Solid Edge part; units mm, degrees
sketch "Sketch1" plane through (0, 0, 0) normal (0, 0, 1) x (1, 0, 0)
  line L0 (-65, 148.37) -> (-65, 118.37)
  line L1 (-65, 118.37) -> (-10, 30)
  line L2 (-10, 30) -> (-10, 0)
  line L3 (-10, 0) -> (0, 0)
  line L4 (0, 0) -> (0, 30)
  line L5 (0, 30) -> (-55, 118.37)
  line L6 (-55, 118.37) -> (-55, 148.37)
  line L7 (-55, 148.37) -> (-65, 148.37)
  dimension "D1" = 55
  dimension "D2" = 10
  dimension "D3" = 55
extrude "Protrusion1" add sketch "Sketch1" against normal blind 30
sketch "Sketch2" plane through (-55, 32.2656, -20) normal (1, 0, 0) x (0, 1, 0)
  circle A0 centre (101.1044, 5) radius 13.5
extrude "Cutout1" cut sketch "Sketch2" against normal up to next
sketch "Sketch3" plane through (0, 15, -15) normal (1, 0, 0) x (0, 0, -1)
  circle A0 centre (0, 0) radius 10
extrude "Cutout2" cut sketch "Sketch3" against normal up to next
Source: CAD feature listing. Evaluate the final solid. Frame: model axes, mm. A direction names the side the tool comes from. Give positions to 0.01 mm unless a question says otherwise; leave off trailing zeros. Order: outer loops, then holes, each group sorted by start corner. A loop starts at its lowest first (then second) coordinate and runs counter-clockwise, first axis right, second up.
(1) Access query for faces 1 (the face through (-65, 134, -1)), 2 (the face through (-10, 15.2, -4.8)), 3 (the face through (-55, 133, -1)). Directions: +Z, -Z, +X, -X, +Y, -Y. A direction counts if a zero-diameter tool reaches every point of the face in a straight line with its end or side. Return the directions, or none.
(2) Material intervals for line 1 along Z through (x, y) = (-60, 133); line 2 along Y through (x, z) = (-3.5, -15); line 3 along Y through (x, z) = (-4, -15), sorted ascending.
(3) Section query C-C (y = 133.37). Return the cut outline in (x, z), plus the area to 3 significant figures.
(4) Pull-direction query (Y, two-part tool) for faces 4 (the face through (-59.93, 146.247, -10.945)), 5 (the face through (-37.885, 74.804, -14.79)), 6 (the face through (-60, 148.37, -15)); classes: +Y half, -Y half, draft (parallel to the pull), parting line (faces both ways), or undercut.
(5) Section query B-B (z = -11.5). Return the cut outline in (x, y).
(6) Contact query for flat-ended pins moving along their axis: P1, Ø2, axis at x = -39, y = 88, coming from the +Z side; P2, Ø6, axis at y = 93, z = -3, coming from the +X side; P3, Ø5, axis at x = -40, z = -7, coming from the -Y side (3 decimals); P4, Ø15, axis at y = 8.5, z = -15, coming from the -X side. Output: stop coordinate, or through.
(7) Section query D-D (x = -6). Return the cut outline in (y, z).
(8) Section query A-A (y = 21). Return the cut outline in (x, z), plus the area to 3 significant figures.
Outcome:
1. face 1: +Z, -Z, -X, +Y, -Y
1. face 2: +Z, -Z, -X, -Y
1. face 3: +Z, -Z, +X, +Y
2. line 1: z = -30 to -28.49, -1.51 to 0
2. line 2: y = 0 to 5, 25 to 35.62
2. line 3: y = 0 to 5, 25 to 36.43
3. outline: (-65, -30) - (-55, -30) - (-55, -28.5) - (-65, -28.5) - close; (-65, -1.5) - (-55, -1.5) - (-55, 0) - (-65, 0) - close
3. area: 30.0 mm2
4. face 4: undercut
4. face 5: -Y half
4. face 6: +Y half
5. outline: (-65, 118.37) - (-10, 30) - (-10, 24.37) - (0, 24.37) - (0, 30) - (-55, 118.37) - (-55, 120.33) - (-65, 120.33) - close; (-65, 146.41) - (-55, 146.41) - (-55, 148.37) - (-65, 148.37) - close; (-10, 0) - (0, 0) - (0, 5.63) - (-10, 5.63) - close
6. P1: stops at z = 0
6. P2: stops at x = -37.34
6. P3: stops at y = 74.185
6. P4: stops at x = -10
7. outline: (0, -30) - (39.64, -30) - (39.64, 0) - (0, 0) - close; hole circle Ø20 at (15, -15)
8. outline: (-10, -30) - (0, -30) - (0, -23) - (-10, -23) - close; (-10, -7) - (0, -7) - (0, 0) - (-10, 0) - close
8. area: 140 mm2
